Design review of the part built by this model. Coordinates are the model's own, in mm. A direction names the side the tool comes from. Round coordinates to 2 decimals unless told otherwise and drop trailing zeros. Loops run counter-clockwise (first coordinate to the right, second up) from the corner with the lowest first, then second, coordinate; pieces in that order, holes last. Notation, with made-up numbers: (-24, 87) - (18, 87) arc R17 ccw to (18, 111) - close; hole circle Ø3 at (38, 6.25). An arc over 180 degrees is marked (long way). One line per question, with ' | ' between items. Start each with the question number.
from build123d import *

# Parameters (mm, degrees)
F3_R      = 1.5
F3_W      = 3.5
F3_H      = 12.5
F4_DEPTH  = 6.5
F5_R      = 1.5
F6_DEPTH  = 4
F7_DEPTH  = 2.5
F8_DEPTH  = 4
F5_W      = 1.25
F5_H      = 1.5
F9_DEPTH  = 25
F10_W     = 3
F10_H     = 1
F11_DEPTH = 0.6
F12_DEPTH = 0.5


with BuildPart() as f4:
    # F3 (on offset) → F4 (new body)
    with BuildSketch(Plane.YZ.offset(4)):
        Polygon((-15.25, 0), (-9, 0), (-9, 12.5), (-15.25, 12.5), (-19, 8.75), (-19, 3.75), align=None)
        with Locations((-15, 6.25)):
            Circle(F3_R, mode=Mode.SUBTRACT)
        with Locations((-7.25, 6.25)):
            Rectangle(F3_W, F3_H)
        with BuildLine():
            Line((5.5, 0), (13, 0))
            Line((13, 0), (13, 12.5))
            Line((13, 12.5), (5.5, 12.5))
            Line((5.5, 12.5), (9.911765, 10.147059))
            ThreePointArc((9.911765, 10.147059), (11.5, 7.5), (9.911765, 4.852941))
            Line((9.911765, 4.852941), (5.5, 2.5))
            Line((5.5, 2.5), (5.5, 0))
        make_face()
        Polygon((13, 12.5), (13, 0), (19.25, 0), (23, 3.75), (23, 8.75), (19.25, 12.5), align=None)
        with Locations((19, 6.25)):
            Circle(F3_R, mode=Mode.SUBTRACT)
    extrude(amount=F4_DEPTH)

    # F5 (on offset) → F6 (join, through all)
    with BuildSketch(Plane.YZ.offset(4)):
        with BuildLine():
            Line((-5.75, 10), (-5.75, 12.5))
            Line((-5.75, 12.5), (-9, 12.5))
            Line((-9, 12.5), (-9, 0))
            Line((-9, 0), (13, 0))
            Line((13, 0), (13, 12.5))
            Line((13, 12.5), (5.75, 12.5))
            Line((5.75, 12.5), (5.75, 10))
            Line((5.75, 10), (5.75, 8.5))
            Line((5.75, 8.5), (4.5, 8.5))
            Line((4.5, 8.5), (0.509121, 6.139305))
            ThreePointArc((0.509121, 6.139305), (0, 6), (-0.509121, 6.139305))
            Line((-0.509121, 6.139305), (-4.5, 8.5))
            Line((-4.5, 8.5), (-5.75, 8.5))
            Line((-5.75, 8.5), (-5.75, 10))
        make_face()
        with Locations((8.5, 7.5)):
            Circle(F5_R, mode=Mode.SUBTRACT)
        Polygon((5.75, 12.5), (-5.75, 12.5), (-5.75, 10), (-4.5, 10), (4.5, 10), (5.75, 10), align=None)
        with BuildLine():
            Line((4.5, 10), (-4.5, 10))
            Line((-4.5, 10), (-4.5, 8.5))
            Line((-4.5, 8.5), (-0.509121, 6.139305))
            ThreePointArc((-0.509121, 6.139305), (0, 6), (0.509121, 6.139305))
            Line((0.509121, 6.139305), (4.5, 8.5))
            Line((4.5, 8.5), (4.5, 10))
        make_face()
    extrude(amount=-F6_DEPTH)

    # F5 (on offset) → F7 (cut)
    with BuildSketch(Plane.YZ.offset(4)):
        with BuildLine():
            Line((4.5, 10), (-4.5, 10))
            Line((-4.5, 10), (-4.5, 8.5))
            Line((-4.5, 8.5), (-0.509121, 6.139305))
            ThreePointArc((-0.509121, 6.139305), (0, 6), (0.509121, 6.139305))
            Line((0.509121, 6.139305), (4.5, 8.5))
            Line((4.5, 8.5), (4.5, 10))
        make_face()
    extrude(amount=-F7_DEPTH, mode=Mode.SUBTRACT)

    # F3 (on offset) → F8 (cut)
    with BuildSketch(Plane.YZ.offset(4)):
        Polygon((-15.25, 0), (-9, 0), (-9, 12.5), (-15.25, 12.5), (-19, 8.75), (-19, 3.75), align=None)
        with Locations((-15, 6.25)):
            Circle(F3_R, mode=Mode.SUBTRACT)
        Polygon((13, 12.5), (13, 0), (19.25, 0), (23, 3.75), (23, 8.75), (19.25, 12.5), align=None)
        with Locations((19, 6.25)):
            Circle(F3_R, mode=Mode.SUBTRACT)
    extrude(amount=F8_DEPTH, mode=Mode.SUBTRACT)

    # F5 (on offset) → F9 (cut)
    with BuildSketch(Plane.YZ.offset(4)):
        Polygon((5.75, 12.5), (-5.75, 12.5), (-5.75, 10), (-4.5, 10), (4.5, 10), (5.75, 10), align=None)
        with Locations((-5.125, 9.25)):
            Rectangle(F5_W, F5_H)
    extrude(amount=F9_DEPTH, mode=Mode.SUBTRACT)

    # F10 (on face) → F11 (cut)
    with BuildSketch(Plane(origin=(0, 0, 0), x_dir=(0, -1, 0), z_dir=(-1, 0, 0))):
        Polygon((-10.5, 12), (-11.5, 12), (-11.5, 11), (-12.5, 11), (-12.5, 10), (-11.5, 10), (-11.5, 9), (-10.5, 9), (-10.5, 10), (-9.5, 10), (-9.5, 11), (-10.5, 11), align=None)
        with Locations((-11, 1)):
            Rectangle(F10_W, F10_H)
    extrude(amount=-F11_DEPTH, mode=Mode.SUBTRACT)

    # F0 (on Right) → F12 (cut)
    with BuildSketch(Plane.YZ):
        with BuildLine():
            Line((-4.5, 8.5), (-5.75, 8.5))
            Line((-5.75, 8.5), (-5.75, 0))
            Line((-5.75, 0), (5.75, 0))
            Line((5.75, 0), (5.75, 8.5))
            Line((5.75, 8.5), (4.5, 8.5))
            Line((4.5, 8.5), (4.5, 10))
            Line((4.5, 10), (5.196152, 10))
            ThreePointArc((5.196152, 10), (0, 13), (-5.196152, 10))
            Line((-5.196152, 10), (-4.5, 10))
            Line((-4.5, 10), (-4.5, 8.5))
        make_face()
    extrude(amount=F12_DEPTH, mode=Mode.SUBTRACT)


solid = f4.part
1. Take a section at D-D, the plane y = -14.5. Give the boundary of the cut face in (x, z).
2. Take a section at C-C, the plane y = 18. Give the boundary of the cut face in (x, z).
3. To check wall thickness, follow line 1 along Z through (x, y) = (9.75, 19); line 2 along Y through (x, z) = (4.5, 11); line 3 along X through (y, z) = (13.5, 3.5). State the ranges of each line that lie inside material, in increasing order.
4. Clearance check with flat-ended pins moving along their axes: P1, Ø2, axis at y = 0.5, z = 8, coming from the -X side; P2, Ø5, axis at y = -15, z = 6, coming from the -X side; P3, Ø0.5, axis at x = 0.5, z = 9.5, coming from the -Y side; P4, Ø5, axis at x = 7, y = 1.5, coming from the -Z side. State where each tip first meets the part, or that it passes through.
5. Take a section at A-A, the plane x = 9.25. Give the boundary of the cut face in (y, z), then the cut area to 3 significant figures.
6. Machinability: for faces 4 (the face through (3, 0, 6)), 5 (the face through (1, -4.5, 9)), 6 (the face through (0.2, 5.75, 7.6)), which of the approach directions +Z, -Z, +X, -X, +Y, -Y give a long, thin tool a straight path to every point of the face, cutting with its end or side? Answer none if there is none.
7. Take a section at B-B, the plane x = 7. Give the boundary of the cut face in (y, z), then the cut area to 3 significant figures.
8. The part is to be moulded in two halves that separate along Z. For faces 1 (the face through (0.5, 0, 6)), 2 (the face through (9.23, 21.15, 10.6)), 3 (the face through (3, -5, 8.5)), say which applies: pulls with the +Z half, pulls with the -Z half, needs draft (parallel to the pull), parting line crosses it, or undercut.
Answer list:
1) outline: (8, 0) - (10.5, 0) - (10.5, 4.84) - (8, 4.84) - close; (8, 7.66) - (10.5, 7.66) - (10.5, 12.5) - (8, 12.5) - close
2) outline: (8, 0) - (10.5, 0) - (10.5, 5.13) - (8, 5.13) - close; (8, 7.37) - (10.5, 7.37) - (10.5, 12.5) - (8, 12.5) - close
3) line 1: z = 0 to 4.75, 7.75 to 12.5 | line 2: y = -9 to -5.75, 8.31 to 13 | line 3: x = 8 to 10.5
4) P1: stops at x = 0.5 | P2: stops at x = 8 | P3: stops at y = -9 | P4: passes through
5) outline: (-19, 3.75) - (-15.25, 0) - (-5.5, 0) - (-5.5, 8.5) - (-5.75, 8.5) - (-5.75, 12.5) - (-15.25, 12.5) - (-19, 8.75) - close; (5.5, 0) - (19.25, 0) - (23, 3.75) - (23, 8.75) - (19.25, 12.5) - (5.75, 12.5) - (5.75, 12.37) - (9.91, 10.15) arc R3 cw to (9.91, 4.85) - (5.5, 2.5) - close; hole circle Ø3 at (-15, 6.25); hole circle Ø3 at (19, 6.25) | area: 304 mm²
6) face 4: +X | face 5: +X, -X | face 6: -X
7) outline: (-9, 0) - (-5.5, 0) - (-5.5, 8.5) - (-5.75, 8.5) - (-5.75, 12.5) - (-9, 12.5) - close; (5.5, 0) - (13, 0) - (13, 12.5) - (5.75, 12.5) - (5.75, 12.37) - (9.91, 10.15) arc R3 cw to (9.91, 4.85) - (5.5, 2.5) - close | area: 96.8 mm²
8) face 1: needs draft | face 2: pulls with the +Z half | face 3: undercut
